Work out the finished part from the listing and answer in its coordinate system (mm). A direction names the side the tool comes from. Round coordinates to 2 decimals unless told otherwise and drop trailing zeros. Write each loop counter-clockwise with the first axis right and the second up, starting at its lowest first coordinate (ties: lowest second). Pieces come first, ordered by that corner, then holes. Notation, with made-up numbers: M -9,-9.75 L 27,-9.75 A10 ccw 27,0.25 Z; hole C 12.5,89 d10. An arc over 180 degrees is marked long. Answer in a Markdown table with one row per item.
```python
from build123d import *

# Parameters (mm, degrees)
SKIZZE4_R                        = 1.75
SCHNITT_LINEAR_AUSTRAGEN2_DEPTH  = 32.670175244
SCHNITT_LINEAR_AUSTRAGEN3_DEPTH  = 4
SKIZZE6_R                        = 1.75
SCHNITT_LINEAR_AUSTRAGEN6_DEPTH  = 32.670175244
FASE1_SIZE                       = 0.5
FASE2_SIZE                       = 0.5
SKIZZE8_W                        = 1.5
SKIZZE8_H                        = 2
SKIZZE8_W_2                      = 2
SKIZZE8_H_2                      = 1.5
SCHNITT_LINEAR_AUSTRAGEN8_DEPTH  = 4
SKIZZE9_R                        = 6
SCHNITT_LINEAR_AUSTRAGEN9_DEPTH  = 32.670175244
SKIZZE11_R                       = 3
SCHNITT_LINEAR_AUSTRAGEN10_DEPTH = 3


with BuildPart() as part:
    # Skizze1 → Rotation1 (revolve)
    with BuildSketch(Plane(origin=(0, 0, 0), x_dir=(0, 0, -1), z_dir=(1, 0, 0)), mode=Mode.PRIVATE) as rotation1_sk:
        Polygon((0, 0), (0, 21), (5, 21), (5, 14), (7.5, 14), (7.5, 12.35), (11, 12.35), (11, 0), align=None)
    revolve(rotation1_sk.sketch.rotate(Axis((0, 0, 0), (0, 0, -1)), 180), axis=Axis((0, 0, 0), (0, 0, -1)))

    # Skizze4 → Schnitt-Linear austragen2 (cut, through all)
    with BuildSketch(Plane.XY):
        with Locations((0, 18)):
            Circle(SKIZZE4_R)
        with Locations((9, 15.588457268)):
            Circle(SKIZZE4_R)
        with Locations((15.588457268, 9)):
            Circle(SKIZZE4_R)
        with Locations((18, 0)):
            Circle(SKIZZE4_R)
        with Locations((15.588457268, -9)):
            Circle(SKIZZE4_R)
        with Locations((9, -15.588457268)):
            Circle(SKIZZE4_R)
        with Locations((0, -18)):
            Circle(SKIZZE4_R)
        with Locations((-9, -15.588457268)):
            Circle(SKIZZE4_R)
        with Locations((-15.588457268, -9)):
            Circle(SKIZZE4_R)
        with Locations((-18, 0)):
            Circle(SKIZZE4_R)
        with Locations((-15.588457268, 9)):
            Circle(SKIZZE4_R)
        with Locations((-9, 15.588457268)):
            Circle(SKIZZE4_R)
    extrude(amount=-SCHNITT_LINEAR_AUSTRAGEN2_DEPTH, mode=Mode.SUBTRACT)

    # Skizze5 → Schnitt-Linear austragen3 (cut)
    with BuildSketch(Plane(origin=(0, 0, -5), x_dir=(-1, 0, 0), z_dir=(0, 0, -1))):
        Polygon((7.41228676, 12.838457268), (10.58771324, 12.838457268), (12.175426481, 15.588457268), (10.58771324, 18.338457268), (7.41228676, 18.338457268), (5.824573519, 15.588457268), align=None)
        Polygon((0, 14.824573519), (2.75, 16.41228676), (2.75, 19.58771324), (0, 21.175426481), (-2.75, 19.58771324), (-2.75, 16.41228676), align=None)
        Polygon((12.838457268, 7.41228676), (15.588457268, 5.824573519), (18.338457268, 7.41228676), (18.338457268, 10.58771324), (15.588457268, 12.175426481), (12.838457268, 10.58771324), align=None)
        Polygon((14.824573519, 0), (16.41228676, -2.75), (19.58771324, -2.75), (21.175426481, 0), (19.58771324, 2.75), (16.41228676, 2.75), align=None)
        Polygon((12.838457268, -7.41228676), (12.838457268, -10.58771324), (15.588457268, -12.175426481), (18.338457268, -10.58771324), (18.338457268, -7.41228676), (15.588457268, -5.824573519), align=None)
        Polygon((7.41228676, -12.838457268), (5.824573519, -15.588457268), (7.41228676, -18.338457268), (10.58771324, -18.338457268), (12.175426481, -15.588457268), (10.58771324, -12.838457268), align=None)
        Polygon((0, -14.824573519), (-2.75, -16.41228676), (-2.75, -19.58771324), (0, -21.175426481), (2.75, -19.58771324), (2.75, -16.41228676), align=None)
        Polygon((-7.41228676, -12.838457268), (-10.58771324, -12.838457268), (-12.175426481, -15.588457268), (-10.58771324, -18.338457268), (-7.41228676, -18.338457268), (-5.824573519, -15.588457268), align=None)
        Polygon((-12.838457268, -7.41228676), (-15.588457268, -5.824573519), (-18.338457268, -7.41228676), (-18.338457268, -10.58771324), (-15.588457268, -12.175426481), (-12.838457268, -10.58771324), align=None)
        Polygon((-14.824573519, 0), (-16.41228676, 2.75), (-19.58771324, 2.75), (-21.175426481, 0), (-19.58771324, -2.75), (-16.41228676, -2.75), align=None)
        Polygon((-12.838457268, 7.41228676), (-12.838457268, 10.58771324), (-15.588457268, 12.175426481), (-18.338457268, 10.58771324), (-18.338457268, 7.41228676), (-15.588457268, 5.824573519), align=None)
        Polygon((-7.41228676, 12.838457268), (-5.824573519, 15.588457268), (-7.41228676, 18.338457268), (-10.58771324, 18.338457268), (-12.175426481, 15.588457268), (-10.58771324, 12.838457268), align=None)
    extrude(amount=-SCHNITT_LINEAR_AUSTRAGEN3_DEPTH, mode=Mode.SUBTRACT)

    # Skizze6 → Schnitt-Linear austragen6 (cut, through all)
    with BuildSketch(Plane.XY):
        with Locations((0, 8.5)):
            Circle(SKIZZE6_R)
        with Locations((8.5, 0)):
            Circle(SKIZZE6_R)
        with Locations((0, -8.5)):
            Circle(SKIZZE6_R)
        with Locations((-8.5, 0)):
            Circle(SKIZZE6_R)
    extrude(amount=-SCHNITT_LINEAR_AUSTRAGEN6_DEPTH, mode=Mode.SUBTRACT)

    # Fase1
    fase1_edges = [part.edges().sort_by_distance(p)[0] for p in [
        (0, 12.35, -11),
        (0, 14, -7.5),
        (0, 14, -5),
    ]]
    chamfer(fase1_edges, length=FASE1_SIZE)

    # Fase2
    fase2_edges = [part.edges().sort_by_distance(p)[0] for p in [
        (0, 21, 0),
    ]]
    chamfer(fase2_edges, length=FASE2_SIZE)

    # Skizze8 → Schnitt-Linear austragen8 (cut)
    with BuildSketch(Plane(origin=(0, 0, -5), x_dir=(-1, 0, 0), z_dir=(0, 0, -1))):
        with Locations((0, 21)):
            Rectangle(SKIZZE8_W, SKIZZE8_H)
        Polygon((10.649519053, 16.945508076), (9.350480947, 17.695508076), (10.350480947, 19.427558883), (11.649519053, 18.677558883), align=None)
        Polygon((17.695508076, 9.350480947), (16.945508076, 10.649519053), (18.677558883, 11.649519053), (19.427558883, 10.350480947), align=None)
        with Locations((21, 0)):
            Rectangle(SKIZZE8_W_2, SKIZZE8_H_2)
        Polygon((16.945508076, -10.649519053), (17.695508076, -9.350480947), (19.427558883, -10.350480947), (18.677558883, -11.649519053), align=None)
        Polygon((9.350480947, -17.695508076), (10.649519053, -16.945508076), (11.649519053, -18.677558883), (10.350480947, -19.427558883), align=None)
        with Locations((0, -21)):
            Rectangle(SKIZZE8_W, SKIZZE8_H)
        Polygon((-10.649519053, -16.945508076), (-9.350480947, -17.695508076), (-10.350480947, -19.427558883), (-11.649519053, -18.677558883), align=None)
        Polygon((-17.695508076, -9.350480947), (-16.945508076, -10.649519053), (-18.677558883, -11.649519053), (-19.427558883, -10.350480947), align=None)
        with Locations((-21, 0)):
            Rectangle(SKIZZE8_W_2, SKIZZE8_H_2)
        Polygon((-16.945508076, 10.649519053), (-17.695508076, 9.350480947), (-19.427558883, 10.350480947), (-18.677558883, 11.649519053), align=None)
        Polygon((-9.350480947, 17.695508076), (-10.649519053, 16.945508076), (-11.649519053, 18.677558883), (-10.350480947, 19.427558883), align=None)
    extrude(amount=-SCHNITT_LINEAR_AUSTRAGEN8_DEPTH, mode=Mode.SUBTRACT)

    # Skizze9 → Schnitt-Linear austragen9 (cut, through all)
    with BuildSketch(Plane.XY):
        Circle(SKIZZE9_R)
    extrude(amount=-SCHNITT_LINEAR_AUSTRAGEN9_DEPTH, mode=Mode.SUBTRACT)

    # Skizze11 → Schnitt-Linear austragen10 (cut)
    with BuildSketch(Plane.XY):
        with Locations((0, 8.5)):
            Circle(SKIZZE11_R)
        with Locations((8.5, 0)):
            Circle(SKIZZE11_R)
        with Locations((0, -8.5)):
            Circle(SKIZZE11_R)
        with Locations((-8.5, 0)):
            Circle(SKIZZE11_R)
    extrude(amount=-SCHNITT_LINEAR_AUSTRAGEN10_DEPTH, mode=Mode.SUBTRACT)


solid = part.part
```
1. A tool of negligible diameter and unlimited length cuts with its end or side. For faces 1 (the flat face through (-9, 18.338, -3)), 2 (the flat face through (-1.394, -15.63, -3.028)), 3 (the cylindrical face through (11.5, -0.1, -1.5)), 4 (the cylindrical face through (-6.831, 0.526, -6.944)), from which of +Z, -Z, +X, -X, +Y, -Y can it reach the whole face along a straight path? Write none if from no direction.
Calculated:
| item | result |
|---|---|
| face 1 | -Z, -X |
| face 2 | -Z |
| face 3 | +Z |
| face 4 | +Z, -Z |
2. Given pin 1 (3 mm diameter, centred on x = -7.5, y = 15.5, fed in from -Z); pin 2 (3 mm diameter, centred on x = -8.5, y = 0, fed in from +Z); pin 3 (1.6 mm diameter, centred on x = 1, y = 17.5, fed in from -Z); pin 4 (6 mm diameter, centred on y = -6.5, z = -8.5, fed in from +X), each flat-ended and moving along its own axis, determine where each tip first touches the part or whether it passes through.
Calculated:
| item | result |
|---|---|
| pin 1 | stops at z = -5 |
| pin 2 | passes through |
| pin 3 | stops at z = -1 |
| pin 4 | stops at x = 13.45 |
3. The part is cut by section A-A (z = -8.5). Determine the outline of the cut face in (x, y).
Calculated:
| item | result |
|---|---|
| outline | C 0,0 d24.7; hole C -8.5,0 d3.5; hole C 0,0 d12; hole C 0,-8.5 d3.5; hole C 0,8.5 d3.5; hole C 8.5,0 d3.5 |
4. The part is cut by section B-B (y = -8.5). Count the separate pieces of the cut face and the enclosed holes in it, plus the area to 3 significant figures.
Calculated:
| item | result |
|---|---|
| separate pieces | 4 |
| enclosed holes | 0 |
| area | 213 mm² |
5. Consider line 1 along Y through (x, z) = (8, -1.5); line 2 along Y through (x, z) = (-2, -0.5); line 3 along X through (y, z) = (0.5, -6.5). Determine where each line is inside the solid, lowest interval first. Write a range as from..to.
Calculated:
| item | result |
|---|---|
| line 1 | y = -19.42..-18.34, -12.84..-2.96, 2.96..12.84, 18.34..19.42 |
| line 2 | y = -20.9..-10.74, -6.26..-5.66, 5.66..6.26, 10.74..20.9 |
| line 3 | x = -13.99..-10.18, -6.82..-5.98, 5.98..6.82, 10.18..13.99 |
